Design review of the part shown in the three views and the two pictorial views. Dimensions are in mm from the part's minimum x, y and z. A direction names the side the tool comes from. Give positions to 0.01 mm unless a question says otherwise; leave off trailing zeros. Loops run counter-clockwise (first coordinate to the right, second up) from the corner with the lowest first, then second, coordinate; pieces in that order, holes last. Notation, with made-up numbers: (2.5, 17.25) -> (58.5, 17.25) arc R25 cw to (58.5, 51.25) -> close; hole circle Ø11 at (-1.75, 55.25). An arc over 180 degrees is marked (long way). Use CSV: the item, a comma, the result in double quotes. Start each with the question number.
Item 1: We need section A-A (y = 10). State the section outline as (x, z) points.
Item 2: The part is to be moulded in two halves that separate along Y. For the marked faces 4, 5 and 6, say which applies: +Y half, -Y half, draft (parallel to the pull), parting line (faces both ways), or undercut.
Item 3: Clearance check with flat-ended pins moving along their axes: pin 1 (5 mm diameter, centred on x = 5, z = 20, fed in from -Y); pin 2 (1.5 mm diameter, centred on x = 2.5, z = 6, fed in from -Y); pin 3 (10 mm diameter, centred on y = 71, z = 5, fed in from +X); pin 4 (3 mm diameter, centred on x = 3.5, y = 23.5, fed in from +Z). State where each tip first meets the part, or that it passes through.
Item 4: We need section D-D (z = 22). State the section outline as (x, y) points.
Item 5: Wall thickness on line 1 along Y through (x, z) = (5, 2); line 2 along X through (y, z) = (90, 2.2); line 3 along Y through (x, z) = (5, 3.85): over which ranges is each line inside the solid? List them lowest first. Write a range as from..to.
Item 6: We need section B-B (x = 5.25). State the section outline as (y, z) points.
Item 7: We need section C-C (z = 3). State the section outline as (x, y) points, plus the area to 3 significant figures.
Item 8: For the marked faces 1, 2 and 3, list the 3-axis set-ups (+Z, -Z, +X, -X, +Y, -Y) from which the entire face can be reached by the end or side of a thin tool; tool diameter is ignored.
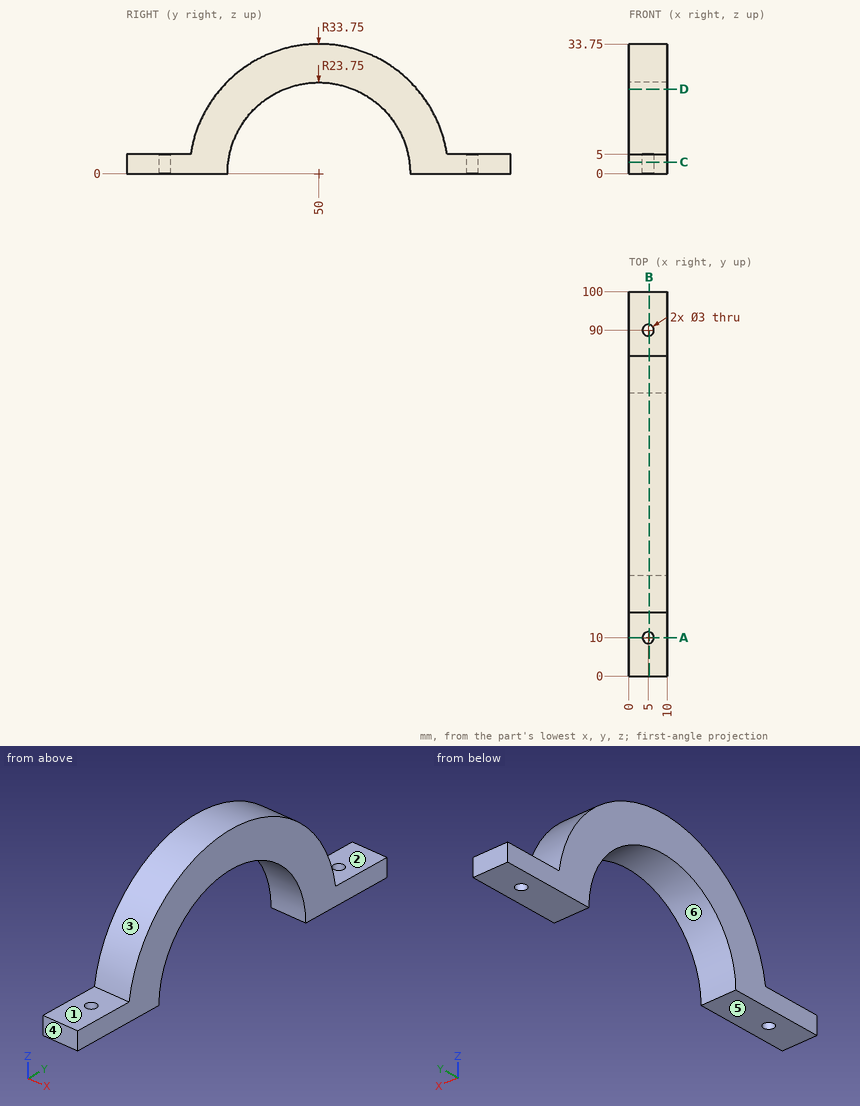
Results found:
1,outline,"(0, 0) -> (3.5, 0) -> (3.5, 5) -> (0, 5) -> close; (6.5, 0) -> (10, 0) -> (10, 5) -> (6.5, 5) -> close"
2,face 4,"-Y half"
2,face 5,"draft"
2,face 6,"undercut"
3,pin 1,"y = 21.14"
3,pin 2,"y = 16.66"
3,pin 3,"x = 10"
3,pin 4,"z = 22.67"
4,outline,"(0, 24.41) -> (10, 24.41) -> (10, 41.05) -> (0, 41.05) -> close; (0, 58.95) -> (10, 58.95) -> (10, 75.59) -> (0, 75.59) -> close"
5,line 1,"0..8.5, 11.5..26.33, 73.67..88.5, 91.5..100"
5,line 2,"0..3.5, 6.5..10"
5,line 3,"0..8.5, 11.5..26.56, 73.44..88.5, 91.5..100"
6,outline,"(0, 0) -> (8.52, 0) -> (8.52, 5) -> (0, 5) -> close; (11.48, 0) -> (26.25, 0) arc R23.75 cw to (73.75, 0) -> (88.52, 0) -> (88.52, 5) -> (83.38, 5) arc R33.75 ccw to (16.62, 5) -> (11.48, 5) -> close; (91.48, 0) -> (100, 0) -> (100, 5) -> (91.48, 5) -> close"
7,outline,"(0, 0) -> (10, 0) -> (10, 26.44) -> (0, 26.44) -> close; (0, 73.56) -> (10, 73.56) -> (10, 100) -> (0, 100) -> close; hole circle Ø3 at (5, 10); hole circle Ø3 at (5, 90)"
7,area,"515 mm²"
8,face 1,"+Z, +X, -X, -Y"
8,face 2,"+Z, +X, -X, +Y"
8,face 3,"+Z, +X, -X"
